from build123d import *

# Parameters (mm, degrees)
F1_DEPTH = 1


with BuildPart() as f1:
    # F0 (on Top) → F1 (new body)
    with BuildSketch(Plane.XY):
        with BuildLine():
            ThreePointArc((7.244152, 7.851622), (25.336024, 9.417542), (41.653382, 1.448117))
            ThreePointArc((41.653382, 1.448117), (48.703058, 1.997731), (48.153443, 9.047407))
            ThreePointArc((48.153443, 9.047407), (37.776237, 23.862356), (36.465034, 41.902585))
            ThreePointArc((36.465034, 41.902585), (32.493609, 47.878818), (26.638178, 43.731348))
            ThreePointArc((26.638178, 43.731348), (18.924994, 27.370544), (3.913004, 17.280485))
            ThreePointArc((3.913004, 17.280485), (0.864147, 10.90048), (7.244152, 7.851622))
        make_face()
        Polygon((28.871957, 24.314205), (31.624682, 20.971675), (30.10633, 16.91648), (25.835252, 16.203815), (23.082526, 19.546344), (24.600879, 23.601539), align=None, mode=Mode.SUBTRACT)
    extrude(amount=F1_DEPTH)


solid = f1.part
For this review, take the finished solid that the model builds, in its own axes (mm). A direction names the side the tool comes from. Coordinates: 2 decimals unless noted, no trailing zeros. Loops run counter-clockwise (first coordinate to the right, second up) from the corner with the lowest first, then second, coordinate; pieces in that order, holes last. Notation, with made-up numbers: (32, -9) - (50, -9) arc R15 ccw to (50, 6) - close; hole circle Ø11 at (-4.75, -36). An arc over 180 degrees is marked (long way). Return JSON: item names as keys, results as strings.
Item 1: Insertion check: pin 1 (3 mm diameter, centred on x = 24.5, y = 27, fed in from -Z). The pin has a flat end and moves straight along its axis. Give the tip position at first contact, or say it passes through.
Determined:
{"pin 1": "stops at z = 0"}
Item 2: Mouldability with a two-part tool opening along Y and no side actions: class faces 1 (the flat face through (30.2, 22.7, 0.5)), 2 (the cylindrical face through (25.083, 9.464, 0.493)), 3 (the flat face through (25, 24, 0)) as pulls with the +Y half, pulls with the -Y half, needs draft (parallel to the pull), parting line crosses it, or undercut.
Determined:
{"face 1": "undercut", "face 2": "pulls with the -Y half", "face 3": "needs draft"}
Item 3: For faces 4 (the flat face through (25, 24, 1)), 5 (the flat face through (24.48, 17.85, 0.49)), list the 3-axis set-ups (+Z, -Z, +X, -X, +Y, -Y) from which the entire face can be reached by the end or side of a thin tool; tool diameter is ignored.
Determined:
{"face 4": "+Z, +X, -X, +Y, -Y", "face 5": "+Z, -Z"}
Item 4: Take a section at B-B (z = 0.2). Give the boundary of the cut face in (x, y), then the cut area to 3 significant figures.
Determined:
{"outline": "(3.91, 17.28) arc R5 ccw to (7.24, 7.85) arc R34 cw to (41.65, 1.45) arc R5 ccw to (48.15, 9.05) arc R34 cw to (36.47, 41.9) arc R5 ccw (long way) to (26.64, 43.73) arc R34 cw to start; hole (23.08, 19.55) - (25.84, 16.2) - (30.11, 16.92) - (31.62, 20.97) - (28.87, 24.31) - (24.6, 23.6) - close", "area": "904 mm2"}
Item 5: Take a section at D-D (y = 27). Give the boundary of the cut face in (x, z), then the cut area to 3 significant figures.
Determined:
{"outline": "(18.6, 0) - (36.83, 0) - (36.83, 1) - (18.6, 1) - close", "area": "18.2 mm2"}
Item 6: Take a section at C-C (x = 39). Give the boundary of the cut face in (y, z).
Determined:
{"outline": "(3.57, 0) - (20.88, 0) - (20.88, 1) - (3.57, 1) - close"}
Item 7: For line 1 (X direction, y = 17, z = 0.55); line 2 (X direction, y = 19, z = 0.25); line 3 (X direction, y = 43.5, z = 0.7), list the stretches that pass through material, from the lowest coordinate up.
Determined:
{"line 1": "x = 3.27 to 25.18, 30.14 to 41.13", "line 2": "x = 8.11 to 23.53, 30.89 to 39.95", "line 3": "x = 26.6 to 36.55"}
Item 8: Take a section at A-A (y = 18.5). Give the boundary of the cut face in (x, z).
Determined:
{"outline": "(7.04, 0) - (23.94, 0) - (23.94, 1) - (7.04, 1) - close; (30.7, 0) - (40.23, 0) - (40.23, 1) - (30.7, 1) - close"}
